Design review of the part built by this model. Coordinates are the model's own, in mm. A direction names the side the tool comes from. Coordinates: 2 decimals unless noted, no trailing zeros. Loops run counter-clockwise (first coordinate to the right, second up) from the corner with the lowest first, then second, coordinate; pieces in that order, holes last. Notation, with made-up numbers: M 31,20.25 L 63,20.25 A27 ccw 63,50.25 Z; hole C -4,84.25 d6. An arc over 180 degrees is marked long. Answer as CSV lines item,"result". Start each with the question number.
from build123d import *

# Parameters (mm, degrees)
SKETCH1_W                 = 40.132
SKETCH1_H                 = 34.29
BOSS_EXTRUDE1_DEPTH       = 20.066
BOSS_EXTRUDE2_DEPTH       = 3.683
SKETCH3_R                 = 6.9215
BOSS_EXTRUDE3_DEPTH       = 1.905
SKETCH4_R                 = 5.08
BOSS_EXTRUDE4_DEPTH       = 0.508
F_6_32_TAPPED_HOLE1_D     = 2.7051
F_6_32_TAPPED_HOLE1_DEPTH = 11.176
F_6_32_TAPPED_HOLE1_TIP   = 0.81269403
SKETCH8_W                 = 20.066
SKETCH8_H                 = 2.54
BOSS_EXTRUDE5_DEPTH       = 7.62
SKETCH9_W                 = 20.066
SKETCH9_H                 = 2.54
BOSS_EXTRUDE6_DEPTH       = 7.62
F_6_CLEARANCE_HOLE1_D     = 3.7973
F_6_CLEARANCE_HOLE1_DEPTH = 3.81
F_6_CLEARANCE_HOLE1_TIP   = 1.140824014
FILLET1_R                 = 1.27


with BuildPart() as part:
    # Sketch1 → Boss-Extrude1 (new body)
    with BuildSketch(Plane(origin=(0, 0, 0), x_dir=(0, 0, -1), z_dir=(1, 0, 0))):
        with Locations((20.066, 17.145)):
            Rectangle(SKETCH1_W, SKETCH1_H)
    extrude(amount=BOSS_EXTRUDE1_DEPTH)

    # Sketch2 → Boss-Extrude2 (add)
    with BuildSketch(Plane(origin=(0, 34.29, 0), x_dir=(1, 0, 0), z_dir=(0, 1, 0))):
        with BuildLine():
            Line((0, 33.782), (20.066, 33.782))
            Line((20.066, 33.782), (20.066, 10.033))
            ThreePointArc((20.066, 10.033), (10.033, 0), (0, 10.033))
            Line((0, 10.033), (0, 33.782))
        make_face()
    extrude(amount=BOSS_EXTRUDE2_DEPTH)

    # Sketch3 → Boss-Extrude3 (add)
    with BuildSketch(Plane(origin=(0, 37.973, 0), x_dir=(1, 0, 0), z_dir=(0, 1, 0))):
        with Locations(Location((10.033, 10.033, 0), (0, 0, 90))):
            Circle(SKETCH3_R)
    extrude(amount=BOSS_EXTRUDE3_DEPTH)

    # Sketch4 → Boss-Extrude4 (add)
    with BuildSketch(Plane(origin=(0, 39.878, 0), x_dir=(1, 0, 0), z_dir=(0, 1, 0))):
        with Locations(Location((10.033, 10.033, 0), (0, 0, 270))):
            Circle(SKETCH4_R)
    extrude(amount=BOSS_EXTRUDE4_DEPTH)

    # #6-32 Tapped Hole1
    with Locations(Plane(origin=(0, 40.386, 0), x_dir=(1, 0, 0), z_dir=(0, 1, 0))):
        with Locations((10.033, 10.033)):
            Hole(F_6_32_TAPPED_HOLE1_D / 2, depth=F_6_32_TAPPED_HOLE1_DEPTH)
            with Locations((0, 0, -(F_6_32_TAPPED_HOLE1_DEPTH + F_6_32_TAPPED_HOLE1_TIP / 2))):  # 118° drill point
                Cone(0, F_6_32_TAPPED_HOLE1_D / 2, F_6_32_TAPPED_HOLE1_TIP, mode=Mode.SUBTRACT)

    # Sketch8 → Boss-Extrude5 (add)
    with BuildSketch(Plane.XY):
        with Locations((10.033, 29.21)):
            Rectangle(SKETCH8_W, SKETCH8_H)
    extrude(amount=BOSS_EXTRUDE5_DEPTH)

    # Sketch9 → Boss-Extrude6 (add)
    with BuildSketch(Plane(origin=(0, 0, -40.132), x_dir=(-1, 0, 0), z_dir=(0, 0, -1))):
        with Locations((-10.033, 29.21)):
            Rectangle(SKETCH9_W, SKETCH9_H)
    extrude(amount=BOSS_EXTRUDE6_DEPTH)

    # #6 Clearance Hole1
    with Locations(Plane(origin=(0, 30.48, 0), x_dir=(1, 0, 0), z_dir=(0, 1, 0))):
        with Locations((14.986, -3.81), (5.08, -3.81), (5.08, 43.942), (14.986, 43.942)):
            Hole(F_6_CLEARANCE_HOLE1_D / 2, depth=F_6_CLEARANCE_HOLE1_DEPTH)
            with Locations((0, 0, -(F_6_CLEARANCE_HOLE1_DEPTH + F_6_CLEARANCE_HOLE1_TIP / 2))):  # 118° drill point
                Cone(0, F_6_CLEARANCE_HOLE1_D / 2, F_6_CLEARANCE_HOLE1_TIP, mode=Mode.SUBTRACT)

    # Fillet1
    fillet1_edges = [part.edges().sort_by_distance(p)[0] for p in [
        (10.033, 0, 0),
        (20.066, 0, -20.066),
        (10.033, 0, -40.132),
        (0, 0, -20.066),
        (0, 32.385, -40.132),
        (0, 13.97, -40.132),
        (20.066, 13.97, -40.132),
        (20.066, 32.385, -40.132),
        (20.066, 32.385, 0),
        (20.066, 13.97, 0),
        (0, 32.385, 0),
        (0, 13.97, 0),
        (20.066, 29.21, -47.752),
        (0, 29.21, -47.752),
        (20.066, 29.21, 7.62),
        (0, 29.21, 7.62),
    ]]
    fillet(fillet1_edges, radius=FILLET1_R)


solid = part.part
Item 1: For faces 1 (the face through (10, 32, -40.132)), 2 (the face through (9.73, 38.91, -3.12)), 3 (the face through (0.362, 32.412, -0.382)), 4 (the face through (0.36, 14.79, -39.75)), list the 3-axis set-ups (+Z, -Z, +X, -X, +Y, -Y) from which the entire face can be reached by the end or side of a thin tool; tool diameter is ignored.
Item 2: Add section D-D (z = -20.5). Give the boundary of the cut face in (x, y).
Item 3: Mouldability with a two-part tool opening along X and no side actions: class faces 5 (the face through (10.25, 28.54, -9.94)), 6 (the face through (19.7, 29.23, 7.24)), 7 (the face through (13.466, 40.128, -13.777)) as released by +X, released by -X, zero draft, split by the parting line, or undercut.
Item 4: For pin 1 (4.5 mm diameter, centred on x = 14.986, z = 3.81, fed in from +Y); pin 2 (6 mm diameter, centred on x = 5.08, z = -43.942, fed in from -Y); pin 3 (7 mm diameter, centred on x = 15, z = -35.5, fed in from +Y), all flat-tipped, find the tip position at first contact; note any pin that passes through.
Item 5: Add section A-A (z = 3.81). Give the boundary of the cut face in (x, y), plus the area to 3 significant figures.
Item 6: Add section B-B (y = 31.5). Give the boundary of the cut face in (x, z).
Item 7: For line 1 along Z through (x, y) = (5.08, 29.9); line 2 along Z through (x, y) = (2.25, 6); line 3 along Y through (x, z) = (16.25, 1), list the stretches that pass through material, from the lowest coordinate up. Write a range as from..to.
Item 8: Add section C-C (y = 7). Give the boundary of the cut face in (x, z), plus the area to 3 significant figures.
Response:
1,face 1,"-Z, +X, -X, +Y"
1,face 2,"+Y"
1,face 3,"+Z, -X, +Y"
1,face 4,"-Z, -X, -Y"
2,outline,"M 0,1.27 A1.27 ccw 1.27,0 L 18.8,0 A1.27 ccw 20.07,1.27 L 20.07,37.97 L 0,37.97 Z"
3,face 5,"undercut"
3,face 6,"released by +X"
3,face 7,"split by the parting line"
4,pin 1,"y = 30.48"
4,pin 2,"y = 27.94"
4,pin 3,"y = 37.97"
5,outline,"M 0,27.94 L 3.18,27.94 L 3.18,30.48 L 0,30.48 Z; M 6.98,27.94 L 13.09,27.94 L 13.09,30.48 L 6.98,30.48 Z; M 16.88,27.94 L 20.07,27.94 L 20.07,30.48 L 16.88,30.48 Z"
5,area,"31.7 mm²"
6,outline,"M 0,-38.86 A1.27 ccw 1.27,-40.13 L 18.8,-40.13 A1.27 ccw 20.07,-38.86 L 20.07,-1.27 A1.27 ccw 18.8,0 L 1.27,0 A1.27 ccw 0,-1.27 Z; hole C 10.03,-10.03 d2.71"
7,line 1,"-47.75..-45.84, -42.04..1.91, 5.71..7.62"
7,line 2,"-40.13..0"
7,line 3,"27.94..30.48"
8,outline,"M 0,-38.86 A1.27 ccw 1.27,-40.13 L 18.8,-40.13 A1.27 ccw 20.07,-38.86 L 20.07,-1.27 A1.27 ccw 18.8,0 L 1.27,0 A1.27 ccw 0,-1.27 Z"
8,area,"804 mm²"
